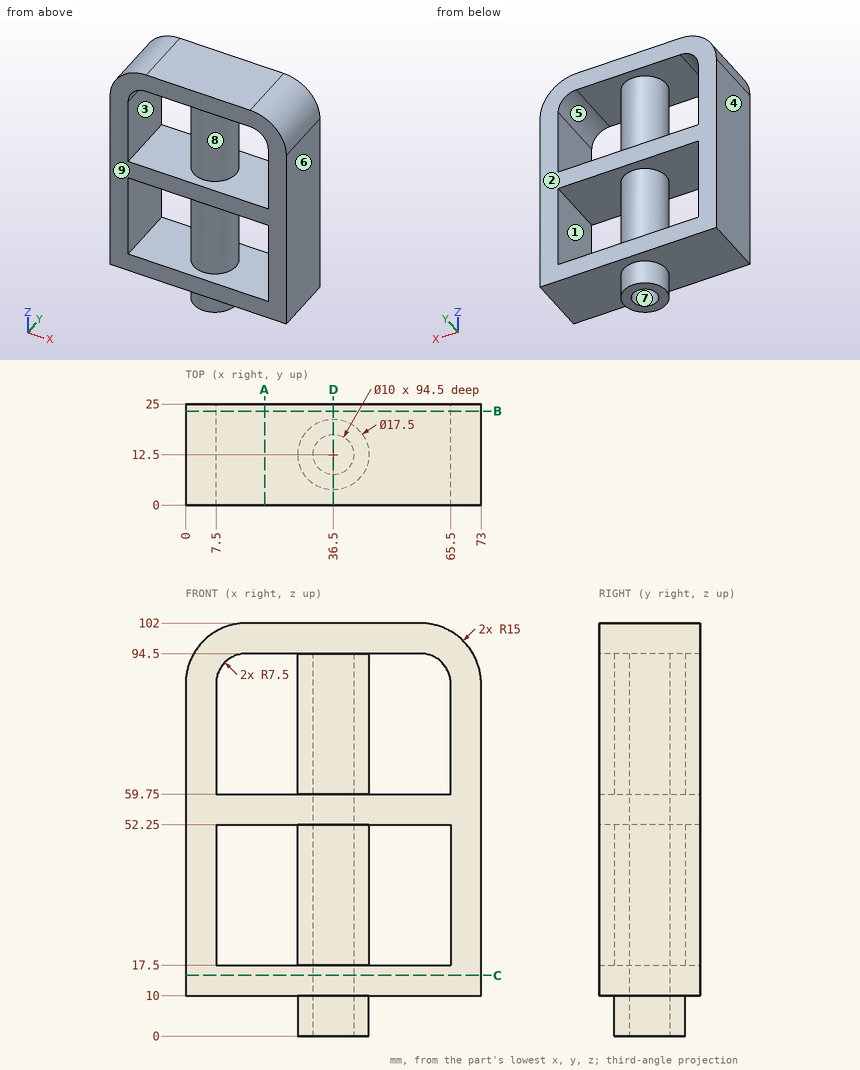
Part print with two shaded views. Sizes in mm from the minimum x, y, z corner. A direction names the side the tool comes from. Round coordinates to 2 decimals unless told otherwise and drop trailing zeros. Order: outer loops, then holes, each group sorted by start corner. A loop starts at its lowest first (then second) coordinate and runs counter-clockwise, first axis right, second up. Notation, with made-up numbers: M -31.75,1.25 L 24.25,1.25 A16 cw 24.25,14.25 Z; hole C 86,36.25 d11. An arc over 180 degrees is marked long. Use CSV: the item, a comma, the result in double quotes. Start each with the question number.
(1) Cut at A-A on x = 19.5. List the corners of the cut face in (y, z).
(2) Tool access for the marked faces 5, 6, 7, 8 and 9: list every direction of +Z, -Z, +X, -X, +Y, -Y with a clear straight run to the whole face (end or side of a thin tool).
(3) Cut at D-D on x = 36.5. List the corners of the cut face in (y, z), then the cut area to 3 significant figures.
(4) Mould opens along X. For the marked faces 1, 2, 3 and 4 say: +X half, -X half, draft (parallel to the pull), parting line (faces both ways), or undercut.
(5) Cut at B-B on y = 23.25. List the corners of the cut face in (x, z).
(6) Drill centre lines: probe 1 along Z at (x, y) = (26, 12); probe 2 along Y at (x, z) = (36.5, 60); probe 3 along Y at (x, z) = (36.5, 52.5). Where is each one in solid material? Low to high.
(7) Flat gauge pin, fed straight in: P1, Ø6, axis at x = 39, z = 78, coming from the -Y side. Where does the tip first touch, or does it go through?
(8) Cut at C-C on z = 15. List the corners of the cut face in (x, y), then the cut area to 3 significant figures.
Findings:
1,outline,"M 0,10 L 25,10 L 25,17.5 L 0,17.5 Z; M 0,52.25 L 25,52.25 L 25,59.75 L 0,59.75 Z; M 0,94.5 L 25,94.5 L 25,102 L 0,102 Z"
2,face 5,"+Y, -Y"
2,face 6,"+Z, -Z, +X, +Y, -Y"
2,face 7,"-Z"
2,face 8,"none"
2,face 9,"+Z, -Z, +X, -X, -Y"
3,outline,"M 0,10 L 3.75,10 L 3.75,0 L 7.5,0 L 7.5,94.5 L 17.5,94.5 L 17.5,0 L 21.25,0 L 21.25,10 L 25,10 L 25,17.5 L 21.25,17.5 L 21.25,52.25 L 25,52.25 L 25,59.75 L 21.25,59.75 L 21.25,94.5 L 25,94.5 L 25,102 L 0,102 L 0,94.5 L 3.75,94.5 L 3.75,59.75 L 0,59.75 L 0,52.25 L 3.75,52.25 L 3.75,17.5 L 0,17.5 Z"
3,area,"1,010 mm^2"
4,face 1,"undercut"
4,face 2,"draft"
4,face 3,"undercut"
4,face 4,"-X half"
5,outline,"M 0,10 L 73,10 L 73,87 A15 ccw 58,102 L 15,102 A15 ccw 0,87 Z; hole M 7.5,17.5 L 65.5,17.5 L 65.5,52.25 L 7.5,52.25 Z; hole M 7.5,59.75 L 65.5,59.75 L 65.5,87 A7.5 ccw 58,94.5 L 15,94.5 A7.5 ccw 7.5,87 Z"
6,probe 1,"z = 10 to 17.5, 52.25 to 59.75, 94.5 to 102"
6,probe 2,"y = 3.75 to 7.5, 17.5 to 21.25"
6,probe 3,"y = 0 to 7.5, 17.5 to 25"
7,P1,"stops at y = 3.75"
8,outline,"M 0,0 L 73,0 L 73,25 L 0,25 Z; hole C 36.5,12.5 d10"
8,area,"1,750 mm^2"
